Read the model definition and answer for the solid it produces. Units are mm, in the model's axes. A direction names the side the tool comes from. Coordinates: 2 decimals unless noted, no trailing zeros. Order: outer loops, then holes, each group sorted by start corner. A loop starts at its lowest first (then second) coordinate and runs counter-clockwise, first axis right, second up. Notation, with made-up numbers: (75, 23.25) - (81, 23.25) arc R5 cw to (81, 27.25) - close; hole circle Ø9 at (4.25, 21). An arc over 180 degrees is marked (long way). Write item = value, one per line.
from build123d import *

# Parameters (mm, degrees)
SKETCH1_W           = 116
SKETCH1_H           = 40
SKETCH1_R           = 5.5
BOSS_EXTRUDE2_DEPTH = 10
SKETCH4_R           = 1
CUT_EXTRUDE1_DEPTH  = 10
SKETCH6_R           = 1
CUT_EXTRUDE3_DEPTH  = 10
SKETCH8_R           = 8.05
CUT_EXTRUDE8_DEPTH  = 5


with BuildPart() as part:
    # Sketch1 → Boss-Extrude2 (new body)
    with BuildSketch(Plane.XY):
        Rectangle(SKETCH1_W, SKETCH1_H)
        Circle(SKETCH1_R, mode=Mode.SUBTRACT)
    extrude(amount=BOSS_EXTRUDE2_DEPTH)

    # Sketch4 → Cut-Extrude1 (cut)
    with BuildSketch(Plane(origin=(58, 0, 0), x_dir=(0, 0, -1), z_dir=(1, 0, 0))):
        with Locations((-5, -5)):
            Circle(SKETCH4_R)
        with Locations((-5, 5)):
            Circle(SKETCH4_R)
    extrude(amount=-CUT_EXTRUDE1_DEPTH, mode=Mode.SUBTRACT)

    # Sketch6 → Cut-Extrude3 (cut)
    with BuildSketch(Plane.ZY.offset(58)):
        with Locations((5, 5)):
            Circle(SKETCH6_R)
        with Locations((5, -5)):
            Circle(SKETCH6_R)
    extrude(amount=-CUT_EXTRUDE3_DEPTH, mode=Mode.SUBTRACT)

    # Sketch8 → Cut-Extrude8 (cut)
    with BuildSketch(Plane.XY):
        Circle(SKETCH8_R)
    extrude(amount=CUT_EXTRUDE8_DEPTH, mode=Mode.SUBTRACT)


solid = part.part
1) The part is cut by section A-A (x = 0). Determine the outline of the cut face in (y, z).
Returned:
outline = (-20, 0) - (-8.05, 0) - (-8.05, 5) - (-5.5, 5) - (-5.5, 10) - (-20, 10) - close; (5.5, 5) - (8.05, 5) - (8.05, 0) - (20, 0) - (20, 10) - (5.5, 10) - close
2) The part is cut by section B-B (y = 3). Determine the outline of the cut face in (x, z), and give its area (3 significant figures).
Returned:
outline = (-58, 0) - (-7.47, 0) - (-7.47, 5) - (-4.61, 5) - (-4.61, 10) - (-58, 10) - close; (4.61, 5) - (7.47, 5) - (7.47, 0) - (58, 0) - (58, 10) - (4.61, 10) - close
area = 1,040 mm^2
3) Determine the mould class of faces 1 (the face through (-1, 9, 0)), 2 (the face through (53, -4, 5)), 3 (the face through (58, 0, 5)) for opening direction Z: pulls with the +Z half, pulls with the -Z half, needs draft (parallel to the pull), parting line crosses it, or undercut.
Returned:
face_1 = pulls with the -Z half
face_2 = undercut
face_3 = needs draft
4) The part is cut by section C-C (z = 3). Determine the outline of the cut face in (x, y), and give its area (3 significant figures).
Returned:
outline = (-58, -20) - (58, -20) - (58, 20) - (-58, 20) - close; hole circle Ø16.1 at (0, 0)
area = 4,440 mm^2
5) For faces 4 (the face through (3, -5, 5)), 5 (the face through (48, 5, 5)), 6 (the face through (-48, 5, 5)), determine the directions among +Z, -Z, +X, -X, +Y, -Y from which every point of the face is accessible in a straight line to the end or side of a thin tool.
Returned:
face_4 = -Z
face_5 = +X
face_6 = -X
6) Straight lines are drawn through the part: line 1 along Y through (x, z) = (-52.25, 5); line 2 along Y through (x, z) = (0, 8.1); line 3 along X through (y, z) = (0, 8.2). For each, find the intervals that lie inside material, in ascending order. Write a range as from..to.
Returned:
line_1 = -20..-6, -4..4, 6..20
line_2 = -20..-5.5, 5.5..20
line_3 = -58..-5.5, 5.5..58
7) Flat-ended cylindrical pins translate along their axes: pin 1 Ø9.5 at (x, y) = (0, 0) entering from +Z; pin 2 Ø0.6 at (y, z) = (5, 5.5) entering from +X; pin 3 Ø1.2 at (y, z) = (-5, 5) entering from -X; pin 4 Ø8 at (x, y) = (2, -2) entering from -Z. Find the tip coordinate at first contact, or state that the pin passes through.
Returned:
pin_1 = through
pin_2 = 48
pin_3 = -48
pin_4 = 5
8) The part is cut by section D-D (y = -7). Determine the outline of the cut face in (x, z).
Returned:
outline = (-58, 0) - (-3.98, 0) - (-3.98, 5) - (3.98, 5) - (3.98, 0) - (58, 0) - (58, 10) - (-58, 10) - close
